The listing builds one solid part. Answer for the finished solid, in the listing's coordinates (mm). Give positions to 0.01 mm unless a question says otherwise; leave off trailing zeros. Write each loop counter-clockwise with the first axis right and the second up, starting at its lowest first coordinate (ties: lowest second). Pieces come first, ordered by that corner, then holes. Notation, with made-up numbers: (54.5, -16.5) -> (106.5, -16.5) arc R27 ccw to (106.5, 22.5) -> close; hole circle Ø4 at (5, 26). An arc over 180 degrees is marked (long way). Use CSV: the item, a comma, the result in double quotes. Start each with the question number.
from build123d import *

# Parameters (mm, degrees)
F1_DEPTH = 12.7
F2_W     = 166.37
F2_H     = 101.854
F3_DEPTH = 10.16
F4_SIZE2 = 3.81
F4_SIZE  = 2.286
F5_R     = 4.572
F6_R     = 1.4605
F7_DEPTH = 10.16
F8_SIZE  = 0.635


with BuildPart() as f1:
    # F0 (on Top) → F1 (new body)
    with BuildSketch(Plane.XY):
        with BuildLine():
            Line((85.598, 61.468), (-85.598, 61.468))
            ThreePointArc((-85.598, 61.468), (-92.7822048969, 58.4922048969), (-95.758, 51.308))
            Line((-95.758, 51.308), (-95.758, -51.308))
            ThreePointArc((-95.758, -51.308), (-92.7822048969, -58.4922048969), (-85.598, -61.468))
            Line((-85.598, -61.468), (85.598, -61.468))
            ThreePointArc((85.598, -61.468), (92.7822048969, -58.4922048969), (95.758, -51.308))
            Line((95.758, -51.308), (95.758, 51.308))
            ThreePointArc((95.758, 51.308), (92.7822048969, 58.4922048969), (85.598, 61.468))
        make_face()
        with BuildLine():
            ThreePointArc((-77.978, 41.148), (-77.2340512242, 42.9440512242), (-75.438, 43.688))
            Line((-75.438, 43.688), (75.438, 43.688))
            ThreePointArc((75.438, 43.688), (77.2340512242, 42.9440512242), (77.978, 41.148))
            Line((77.978, 41.148), (77.978, -41.148))
            ThreePointArc((77.978, -41.148), (77.2340512242, -42.9440512242), (75.438, -43.688))
            Line((75.438, -43.688), (-75.438, -43.688))
            ThreePointArc((-75.438, -43.688), (-77.2340512242, -42.9440512242), (-77.978, -41.148))
            Line((-77.978, -41.148), (-77.978, 41.148))
        make_face(mode=Mode.SUBTRACT)
    extrude(amount=F1_DEPTH)

    # F2 (on face) → F3 (cut)
    with BuildSketch(Plane(origin=(0, 0, 0), x_dir=(1, 0, 0), z_dir=(0, 0, -1))):
        with Locations((1.397, 2.159)):
            Rectangle(F2_W, F2_H)
    extrude(amount=-F3_DEPTH, mode=Mode.SUBTRACT)

    # F4
    f4_edges = [f1.edges().sort_by_distance(p)[0] for p in [
        (0, -43.688, 12.7),
    ]]
    f4_side = f1.faces().sort_by_distance((0, -43.688, 11.43))[0]
    chamfer(f4_edges, length=F4_SIZE, length2=F4_SIZE2, reference=f4_side)

    # F5
    f5_edges = [f1.edges().sort_by_distance(p)[0] for p in [
        (0, -61.468, 12.7),
    ]]
    fillet(f5_edges, radius=F5_R)

    # F6 (on face) → F7 (cut)
    with BuildSketch(Plane(origin=(0, 0, 0), x_dir=(1, 0, 0), z_dir=(0, 0, -1))):
        with Locations((-63.5, 56.134)):
            Circle(F6_R)
        with Locations((63.5, 56.134)):
            Circle(F6_R)
        with Locations((-63.5, -51.816)):
            Circle(F6_R)
        with Locations((63.5, -51.816)):
            Circle(F6_R)
        with Locations((-90.424, 47.625)):
            Circle(F6_R)
        with Locations((-90.424, -47.625)):
            Circle(F6_R)
        with Locations((90.424, -47.625)):
            Circle(F6_R)
        with Locations((90.424, 47.625)):
            Circle(F6_R)
        with Locations((-90.424, 0)):
            Circle(F6_R)
        with Locations((90.424, 0)):
            Circle(F6_R)
        with Locations((-33.02, 56.134)):
            Circle(F6_R)
        with Locations((33.02, 56.134)):
            Circle(F6_R)
        with Locations((-33.02, -56.134)):
            Circle(F6_R)
        with Locations((33.02, -56.134)):
            Circle(F6_R)
    extrude(amount=-F7_DEPTH, mode=Mode.SUBTRACT)

    # F8
    f8_edges = [f1.edges().sort_by_distance(p)[0] for p in [
        (1.397, -53.086, 0),
        (0, -61.468, 0),
        (-81.788, -2.159, 0),
        (1.397, 48.768, 0),
        (84.582, -2.159, 0),
    ]]
    chamfer(f8_edges, length=F8_SIZE)


solid = f1.part
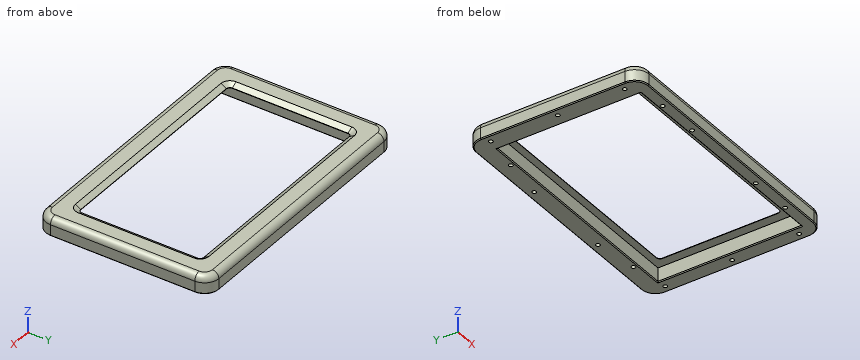
Q1. Section C-C on z = 3 is taken. State how many separate pieces and enclosed holes the cut face has, then the cut area to 3 significant figures.
Q2. Section B-B on x = 57 is taken. Give the vertices of the cut face in (y, z) (3 decimals).
Q3. Flat-ended cylindrical pins translate along their axes: pin 1 Ø1.8 at (x, y) = (90.424, 0) entering from -Z; pin 2 Ø1.5 at (x, z) = (15.5, 9.5) entering from +Y. Find the tip coordinate at first contact, or state that the pin passes through.
Q4. Section A-A on y = -28 is taken. Give the vertices of the cut face in (x, z) (3 decimals), then the cut area to 3 significant figures.
Q5. Straight lines are drawn through the part: L1, parallel to X at y = -4, z = 4.5; L2, parallel to Y at x = -33.02, z = 7; L3, parallel to Y at x = 78.5, z = 3.75. For each, find the intervals that lie inside material, in ascending order.
Output:
1,separate pieces,"1"
1,enclosed holes,"15"
1,area,"6,420 mm²"
2,outline,"(-61.468, 0.635) -> (-60.833, 0) -> (-53.721, 0) -> (-53.086, 0.635) -> (-53.086, 10.16) -> (-43.688, 10.16) -> (-43.688, 10.414) -> (-47.498, 12.7) -> (-56.896, 12.7) arc R4.572 ccw to (-61.468, 8.128) -> close; (43.688, 10.16) -> (48.768, 10.16) -> (48.768, 0.635) -> (49.403, 0) -> (60.833, 0) -> (61.468, 0.635) -> (61.468, 8.128) arc R4.572 ccw to (56.896, 12.7) -> (47.498, 12.7) -> (43.688, 10.414) -> close"
3,pin 1,"z = 10.16"
3,pin 2,"y = 61.43"
4,outline,"(-95.758, 0.635) -> (-95.123, 0) -> (-82.423, 0) -> (-81.788, 0.635) -> (-81.788, 10.16) -> (-77.978, 10.16) -> (-77.978, 10.414) -> (-81.788, 12.7) -> (-91.186, 12.7) arc R4.572 ccw to (-95.758, 8.128) -> close; (77.978, 10.16) -> (84.582, 10.16) -> (84.582, 0.635) -> (85.217, 0) -> (95.123, 0) -> (95.758, 0.635) -> (95.758, 8.128) arc R4.572 ccw to (91.186, 12.7) -> (81.788, 12.7) -> (77.978, 10.414) -> close"
4,area,"327 mm²"
5,L1,"-95.76 to -81.79, 84.58 to 95.76"
5,L2,"-61.47 to -57.59, -54.67 to -53.09, 48.77 to 54.67, 57.59 to 61.47"
5,L3,"-61.47 to -53.09, 48.77 to 61.47"
